Part print with two shaded views. Sizes in mm from the minimum x, y, z corner. A direction names the side the tool comes from. Round coordinates to 2 decimals unless told otherwise and drop trailing zeros. Write each loop counter-clockwise with the first axis right and the second up, starting at its lowest first coordinate (ties: lowest second). Pieces come first, ordered by that corner, then holes. Notation, with made-up numbers: (70, 28.25) - (93, 28.25) arc R18 cw to (93, 53.25) - close; hole circle Ø6 at (16.25, -20). An arc over 180 degrees is marked (long way). Answer as a JSON object with one key per item and string values. Group by question number.
Item 1: Probe line 1 (Z direction, x = 22.5, y = 102); line 2 (X direction, y = 80.5, z = 28); line 3 (X direction, y = 124.5, z = 92). List the from-to ranges inside material, lowest first. Write a range as from..to.
Item 2: Slice it at B-B, the plane z = 82. List the corners of the cut face in (x, y).
Item 3: Which spindle directions (+Z, -Z, +X, -X, +Y, -Y) get a long thin tool onto all of the face, cutting with end or side? Do the marked faces 1, 2 and 3. Say none if no direction does.
Item 4: Slice it at C-C, the plane x = 27. List the corners of the cut face in (y, z).
Item 5: Slice it at D-D, the plane y = 62. List the corners of the cut face in (x, z).
Item 6: Slice it at A-A, the plane y = 34. List the corners of the cut face in (x, z).
Item 7: Flat gauge pins, fed straight in: pin 1 (10 mm diameter, centred on x = 83, y = 67, fed in from +Z); pin 2 (1 mm diameter, centred on y = 133.5, z = 62.5, fed in from -X); pin 3 (3 mm diameter, centred on x = 64.5, z = 154, fed in from +Y). Where does each tip first touch, or does it go through?
Item 8: Two-plate mould, pull along Y, no slides. Class the marked faces 4, 5 and 6: +Y half, -Y half, draft (parallel to the pull), parting line (faces both ways), or undercut.
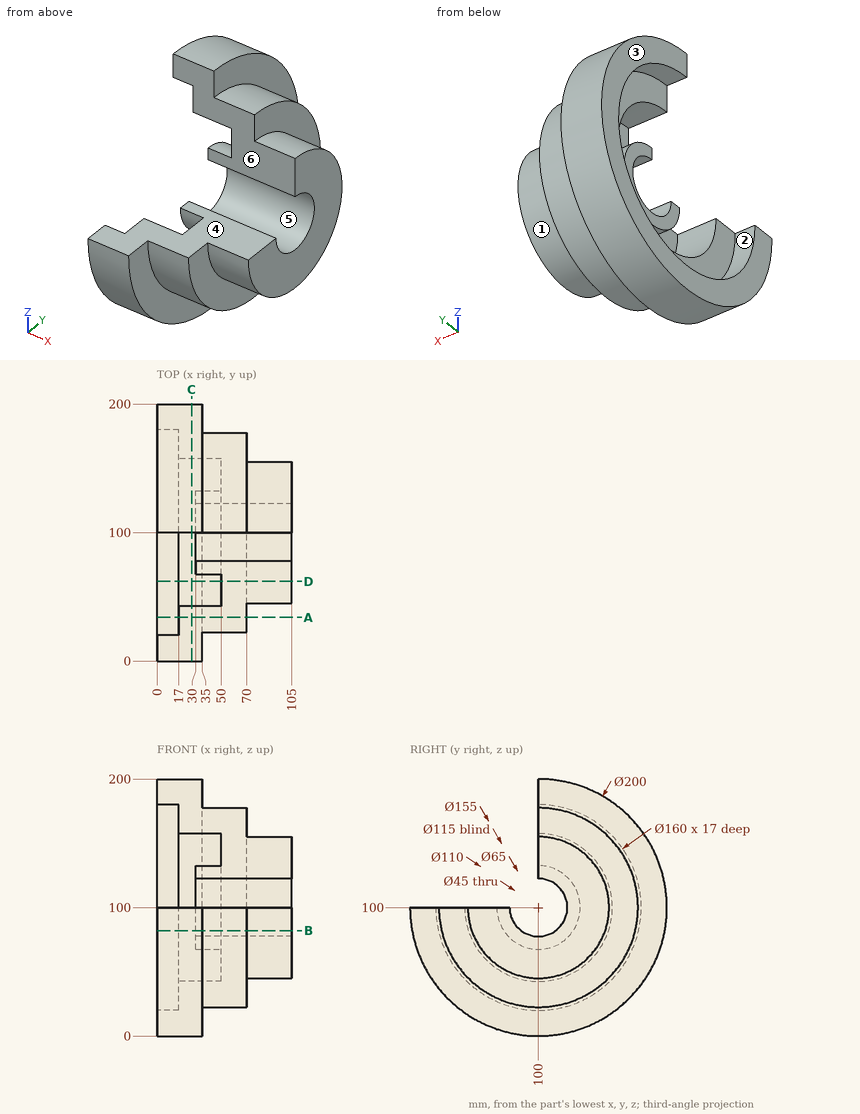
Geometry says:
{
 "1": {"line 1": "z = 0.02..42.53, 157.47..199.98", "line 2": "x = 17..70", "line 3": "x = 30..105"},
 "2": {"outline": "(0, 1.63) - (35, 1.63) - (35, 24.62) - (70, 24.62) - (70, 48.03) - (105, 48.03) - (105, 86.5) - (30, 86.5) - (30, 72.94) - (50, 72.94) - (50, 45.39) - (17, 45.39) - (17, 22.05) - (0, 22.05) - close; (0, 177.95) - (17, 177.95) - (17, 154.61) - (50, 154.61) - (50, 127.06) - (30, 127.06) - (30, 113.5) - (105, 113.5) - (105, 151.97) - (70, 151.97) - (70, 175.38) - (35, 175.38) - (35, 198.37) - (0, 198.37) - close"},
 "3": {"face 1": "+X", "face 2": "-X", "face 3": "+Z, -Z, -X, +Y, -Y"},
 "4": {"outline": "(0, 100) arc R100 ccw (long way) to (100, 200) - (100, 157.5) arc R57.5 cw (long way) to (42.5, 100) - close"},
 "5": {"outline": "(0, 7.5) - (35, 7.5) - (35, 32.46) - (70, 32.46) - (70, 60.24) - (105, 60.24) - (105, 100) - (50, 100) - (50, 56.85) - (17, 56.85) - (17, 29.6) - (0, 29.6) - close"},
 "6": {"outline": "(0, 24.87) - (35, 24.87) - (35, 59.38) - (70, 59.38) - (70, 100) - (17, 100) - (17, 54.79) - (0, 54.79) - close"},
 "7": {"pin 1": "stops at z = 100", "pin 2": "stops at x = 50", "pin 3": "stops at y = 157.01"},
 "8": {"face 4": "draft", "face 5": "undercut", "face 6": "-Y half"}
}
